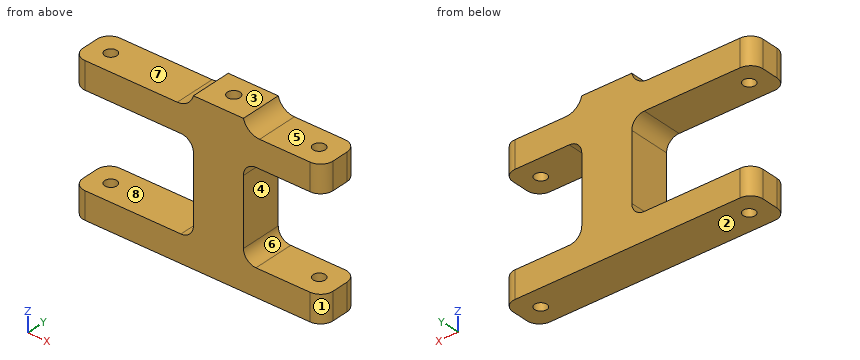
```python
from build123d import *

# Parameters (mm, degrees)
SKETCH1_W               = 60
SKETCH1_H               = 35
BOSS_EXTRUDE1_DEPTH     = 10
SKETCH2_W               = 22
SKETCH2_H               = 10
CUT_EXTRUDE1_DEPTH      = 19
SKETCH3_W               = 22
SKETCH3_H               = 10
CUT_EXTRUDE2_DEPTH      = 29
SKETCH5_R               = 1.45
CUT_EXTRUDE4_DEPTH      = 71.178344238
FILLET1_R               = 3
FILLET2_R               = 3
SKETCH7_W               = 12
SKETCH7_H               = 10
BOSS_EXTRUDE2_DEPTH     = 3
CUT_EXTRUDE5_DEPTH      = 3
CUT_EXTRUDE5_DEPTH_BACK = 15
SKETCH6_R               = 1.5
FILLET3_R               = 4


with BuildPart() as part:
    # Sketch1 → Boss-Extrude1 (new body)
    with BuildSketch(Plane(origin=(0, 0, 0), x_dir=(1, 0, 0), z_dir=(0, 1, 0))):
        with Locations((30, -17.5)):
            Rectangle(SKETCH1_W, SKETCH1_H)
    extrude(amount=BOSS_EXTRUDE1_DEPTH)

    # Sketch2 → Cut-Extrude1 (cut)
    with BuildSketch(Plane(origin=(60, 0, 0), x_dir=(0, 0, -1), z_dir=(1, 0, 0))):
        with Locations((-17.5, 5)):
            Rectangle(SKETCH2_W, SKETCH2_H)
    extrude(amount=-CUT_EXTRUDE1_DEPTH, mode=Mode.SUBTRACT)

    # Sketch3 → Cut-Extrude2 (cut)
    with BuildSketch(Plane.ZY):
        with Locations((17.5, 5)):
            Rectangle(SKETCH3_W, SKETCH3_H)
    extrude(amount=-CUT_EXTRUDE2_DEPTH, mode=Mode.SUBTRACT)

    # Sketch5 → Cut-Extrude4 (cut, through all)
    with BuildSketch(Plane.XY.offset(35)):
        with Locations((5, 5)):
            Circle(SKETCH5_R)
        with Locations((55, 5)):
            Circle(SKETCH5_R)
    extrude(amount=-CUT_EXTRUDE4_DEPTH, mode=Mode.SUBTRACT)

    # Fillet1
    fillet1_edges = [part.edges().sort_by_distance(p)[0] for p in [
        (60, 10, 31.75),
        (60, 0, 3.25),
        (60, 10, 3.25),
        (0, 0, 31.75),
        (0, 10, 31.75),
        (0, 10, 3.25),
        (60, 0, 31.75),
        (0, 0, 3.25),
    ]]
    fillet(fillet1_edges, radius=FILLET1_R)

    # Fillet2
    fillet2_edges = [part.edges().sort_by_distance(p)[0] for p in [
        (41, 5, 28.5),
        (41, 5, 6.5),
        (29, 5, 6.5),
        (29, 5, 28.5),
    ]]
    fillet(fillet2_edges, radius=FILLET2_R)

    # Sketch7 → Boss-Extrude2 (add)
    with BuildSketch(Plane.XY.offset(35)):
        with Locations((35, 5)):
            Rectangle(SKETCH7_W, SKETCH7_H)
    extrude(amount=BOSS_EXTRUDE2_DEPTH)

    # Sketch6 → Cut-Extrude5 (cut, two sides: drawn at the far end of the back side and taken through both)
    with BuildSketch(Plane.XY.offset(35).offset(-CUT_EXTRUDE5_DEPTH_BACK)):
        with Locations((34.5, 5)):
            Circle(SKETCH6_R)
    extrude(amount=CUT_EXTRUDE5_DEPTH + CUT_EXTRUDE5_DEPTH_BACK, mode=Mode.SUBTRACT)

    # Fillet3
    # the kernel refuses this fillet: 4 mm, written as the material it adds along each edge
    with BuildSketch(Plane(origin=(41, 10, 35), x_dir=(0, 0, 1), z_dir=(0, -1, 0))) as fillet3_piece_1:
        with BuildLine():
            CenterArc((4, -3.872983346), FILLET3_R, 104.477512186, 75.522487814)
            Line((0, -3.872983346), (-0.08, -3.872983346))
            Line((-0.08, -3.872983346), (-0.08, 0))
            Line((-0.08, 0), (0, 0.08))
            ThreePointArc((0, 0.08), (1.5, 0.08), (2.98, 0.077459667))
            Line((2.98, 0.077459667), (3, 0))
        make_face()
    extrude(amount=10)
    with BuildSketch(Plane(origin=(29, 0, 35), x_dir=(-1, 0, 0), z_dir=(0, 1, 0))) as fillet3_piece_2:
        with BuildLine():
            CenterArc((3.872983346, 4), FILLET3_R, 194.477512186, 75.522487814)
            Line((0, 3), (-0.077459667, 2.98))
            ThreePointArc((-0.077459667, 2.98), (-0.08, 1.5), (-0.08, 0))
            Line((-0.08, 0), (0, -0.08))
            Line((0, -0.08), (3.872983346, -0.08))
            Line((3.872983346, -0.08), (3.872983346, 0))
        make_face()
    extrude(amount=10)


solid = part.part
```
Geometry: final body of the model. Coordinates: model frame, mm. Face numbers are marked on the shaded views. A direction names the side the tool comes from. Coordinates: 2 decimals unless noted, no trailing zeros. Order: outer loops, then holes, each group sorted by start corner. A loop starts at its lowest first (then second) coordinate and runs counter-clockwise, first axis right, second up. Notation, with made-up numbers: (27.5, 74.5) -> (47.5, 74.5) arc R22 cw to (47.5, 97.5) -> close; hole circle Ø4 at (-6, 80). An arc over 180 degrees is marked (long way). Write item = value, one per line.
(1) Line query: line 1 (Z direction, x = 24, y = 2.25); line 2 (Y direction, x = 55, z = 32.75); line 3 (Y direction, x = 34.5, z = 29.75). Output: solid intervals per line, ascending.
Solved:
line_1 = 0 to 6.5, 28.5 to 35
line_2 = 0 to 3.55, 6.45 to 10
line_3 = 0 to 3.5, 6.5 to 10
(2) Pin query (flat end, axial travel): pin 1 Ø3 at (y, z) = (6.5, 15.5) entering from +X; pin 2 Ø0.9 at (x, y) = (35, 5) entering from +Z; pin 3 Ø3 at (x, y) = (11, 4) entering from +Z. Return the tip coordinate at first contact, or that it passes through.
Solved:
pin_1 = 41
pin_2 = 20
pin_3 = 35
(3) Cut plane C-C on z = 2. Return loops of the section in (x, y).
Solved:
outline = (0, 3) arc R3 ccw to (3, 0) -> (57, 0) arc R3 ccw to (60, 3) -> (60, 7) arc R3 ccw to (57, 10) -> (3, 10) arc R3 ccw to (0, 7) -> close; hole circle Ø2.9 at (5, 5); hole circle Ø2.9 at (55, 5)
(4) Access query for the marked faces 5, 6, 7 and 8. Directions: +Z, -Z, +X, -X, +Y, -Y. A direction counts if a zero-diameter tool reaches every point of the face in a straight line with its end or side. Return the directions, or none.
Solved:
face_5 = +Z, +X, +Y, -Y
face_6 = +X, +Y, -Y
face_7 = +Z, -X, +Y, -Y
face_8 = -X, +Y, -Y
(5) Cut plane D-D on x = 5. Return loops of the section in (y, z), plus the area to 3 significant figures.
Solved:
outline = (0, 0) -> (3.55, 0) -> (3.55, 6.5) -> (0, 6.5) -> close; (0, 28.5) -> (3.55, 28.5) -> (3.55, 35) -> (0, 35) -> close; (6.45, 0) -> (10, 0) -> (10, 6.5) -> (6.45, 6.5) -> close; (6.45, 28.5) -> (10, 28.5) -> (10, 35) -> (6.45, 35) -> close
area = 92.3 mm²
(6) Pull-direction query (Z, two-part tool) for the marked faces 1, 2, 3 and 4; classes: pulls with the +Z half, pulls with the -Z half, needs draft (parallel to the pull), parting line crosses it, or undercut.
Solved:
face_1 = needs draft
face_2 = pulls with the -Z half
face_3 = pulls with the +Z half
face_4 = undercut
(7) Cut plane A-A on z = 30. Return loops of the section in (x, y).
Solved:
outline = (0, 3) arc R3 ccw to (3, 0) -> (57, 0) arc R3 ccw to (60, 3) -> (60, 7) arc R3 ccw to (57, 10) -> (3, 10) arc R3 ccw to (0, 7) -> close; hole circle Ø2.9 at (5, 5); hole circle Ø3 at (34.5, 5); hole circle Ø2.9 at (55, 5)
(8) Cut plane B-B on x = 46. Return loops of the section in (y, z).
Solved:
outline = (0, 0) -> (10, 0) -> (10, 6.5) -> (0, 6.5) -> close; (0, 28.5) -> (10, 28.5) -> (10, 35) -> (0, 35) -> close
